from build123d import *

# Parameters (mm, degrees)
BASE_DEPTH                            = 5
ESQUISSE3_R                           = 2
ESQUISSE3_W                           = 65
ESQUISSE3_H                           = 30
PER_AGE_ROUES_ENCODEUSES_DEPTH        = 6
CONG_1_R                              = 3
PER_AGE_BILLES_PORTEUSES_REACH        = 7
ESQUISSE6_R                           = 2
ESQUISSE6_R_2                         = 11
PER_AGE_PROFIL_S_REACH                = 7
ESQUISSE8_R                           = 3
ESQUISSE15_R                          = 2.2
PER_AGE_BLOC_MOTEUR_DEPTH             = 5
ESQUISSE16_W                          = 65
ESQUISSE16_H                          = 38
ENL_V_MAT_EXTRU_1_DEPTH               = 6
ESQUISSE19_R                          = 1.75
PER_AGE_ACTIONNEUR_MAIN_DE_DIEU_DEPTH = 6


with BuildPart() as part:
    # Esquisse1 → Base (new body)
    with BuildSketch(Plane.XY):
        Polygon((0, 0), (-200, 0), (-224.748737342, 24.748737342), (-224.748737342, 284.748737342), (-200, 309.497474683), (0, 309.497474683), (24.748737342, 284.748737342), (24.748737342, 24.748737342), align=None)
    extrude(amount=BASE_DEPTH)

    # Esquisse3 → Perçage roues encodeuses (cut, through all)
    with BuildSketch(Plane(origin=(0, 0, 0), x_dir=(-1, 0, 0), z_dir=(0, 0, -1))):
        with Locations((65, 45)):
            Circle(ESQUISSE3_R)
        with Locations((135, 45)):
            Circle(ESQUISSE3_R)
        with Locations((135, 264.497474683)):
            Circle(ESQUISSE3_R)
        with Locations((65, 264.497474683)):
            Circle(ESQUISSE3_R)
        Polygon((142, 0), (142, 20), (118, 20), (118, 45.5), (82, 45.5), (82, 20), (58, 20), (58, 0), align=None)
        Polygon((58, 309.497474683), (142, 309.497474683), (142, 289.497474683), (118, 289.497474683), (118, 263.997474683), (82, 263.997474683), (82, 289.497474683), (58, 289.497474683), align=None)
        with Locations((100, 229.497474683)):
            Rectangle(ESQUISSE3_W, ESQUISSE3_H)
        with Locations((100, 80)):
            Rectangle(ESQUISSE3_W, ESQUISSE3_H)
    extrude(amount=-PER_AGE_ROUES_ENCODEUSES_DEPTH, mode=Mode.SUBTRACT)

    # Congé1
    cong_1_edges = [part.edges().sort_by_distance(p)[0] for p in [
        (0, 0, 2.5),
        (-200, 0, 2.5),
        (-224.748737342, 24.748737342, 2.5),
        (-224.748737342, 284.748737342, 2.5),
        (-200, 309.497474683, 2.5),
        (0, 309.497474683, 2.5),
        (24.748737342, 284.748737342, 2.5),
        (24.748737342, 24.748737342, 2.5),
        (-58, 289.497474683, 2.5),
        (-58, 309.497474683, 2.5),
        (-142, 309.497474683, 2.5),
        (-142, 289.497474683, 2.5),
        (-118, 289.497474683, 2.5),
        (-118, 263.997474683, 2.5),
        (-82, 263.997474683, 2.5),
        (-82, 289.497474683, 2.5),
        (-142, 0, 2.5),
        (-58, 0, 2.5),
        (-58, 20, 2.5),
        (-82, 20, 2.5),
        (-82, 45.5, 2.5),
        (-118, 45.5, 2.5),
        (-118, 20, 2.5),
        (-142, 20, 2.5),
    ]]
    fillet(cong_1_edges, radius=CONG_1_R)

    # Esquisse6 → Perçage billes porteuses (cut, up to next)
    with BuildSketch(Plane.XY.offset(5), mode=Mode.PRIVATE) as per_age_billes_porteuses_sk1:
        with Locations((-180.748737342, 28)):
            Circle(ESQUISSE6_R)
    per_age_billes_porteuses_tool1 = extrude(per_age_billes_porteuses_sk1.sketch, amount=-PER_AGE_BILLES_PORTEUSES_REACH, mode=Mode.PRIVATE) & part.part
    add(per_age_billes_porteuses_tool1.solids().sort_by_distance((-180.748737, 28, 5))[0], mode=Mode.SUBTRACT)
    # Esquisse6 → Perçage billes porteuses (cut, up to next)
    with BuildSketch(Plane.XY.offset(5), mode=Mode.PRIVATE) as per_age_billes_porteuses_sk2:
        with Locations((-210.748737342, 28)):
            Circle(ESQUISSE6_R)
    per_age_billes_porteuses_tool2 = extrude(per_age_billes_porteuses_sk2.sketch, amount=-PER_AGE_BILLES_PORTEUSES_REACH, mode=Mode.PRIVATE) & part.part
    add(per_age_billes_porteuses_tool2.solids().sort_by_distance((-210.748737, 28, 5))[0], mode=Mode.SUBTRACT)
    # Esquisse6 → Perçage billes porteuses (cut, up to next)
    with BuildSketch(Plane.XY.offset(5), mode=Mode.PRIVATE) as per_age_billes_porteuses_sk3:
        with Locations((-195.748737342, 28)):
            Circle(ESQUISSE6_R_2)
    per_age_billes_porteuses_tool3 = extrude(per_age_billes_porteuses_sk3.sketch, amount=-PER_AGE_BILLES_PORTEUSES_REACH, mode=Mode.PRIVATE) & part.part
    add(per_age_billes_porteuses_tool3.solids().sort_by_distance((-195.748737, 28, 5))[0], mode=Mode.SUBTRACT)
    # Esquisse6 → Perçage billes porteuses (cut, up to next)
    with BuildSketch(Plane.XY.offset(5), mode=Mode.PRIVATE) as per_age_billes_porteuses_sk4:
        with Locations((-19.251262658, 28)):
            Circle(ESQUISSE6_R)
    per_age_billes_porteuses_tool4 = extrude(per_age_billes_porteuses_sk4.sketch, amount=-PER_AGE_BILLES_PORTEUSES_REACH, mode=Mode.PRIVATE) & part.part
    add(per_age_billes_porteuses_tool4.solids().sort_by_distance((-19.251263, 28, 5))[0], mode=Mode.SUBTRACT)
    # Esquisse6 → Perçage billes porteuses (cut, up to next)
    with BuildSketch(Plane.XY.offset(5), mode=Mode.PRIVATE) as per_age_billes_porteuses_sk5:
        with Locations((10.748737342, 28)):
            Circle(ESQUISSE6_R)
    per_age_billes_porteuses_tool5 = extrude(per_age_billes_porteuses_sk5.sketch, amount=-PER_AGE_BILLES_PORTEUSES_REACH, mode=Mode.PRIVATE) & part.part
    add(per_age_billes_porteuses_tool5.solids().sort_by_distance((10.748737, 28, 5))[0], mode=Mode.SUBTRACT)
    # Esquisse6 → Perçage billes porteuses (cut, up to next)
    with BuildSketch(Plane.XY.offset(5), mode=Mode.PRIVATE) as per_age_billes_porteuses_sk6:
        with Locations((-4.251262658, 28)):
            Circle(ESQUISSE6_R_2)
    per_age_billes_porteuses_tool6 = extrude(per_age_billes_porteuses_sk6.sketch, amount=-PER_AGE_BILLES_PORTEUSES_REACH, mode=Mode.PRIVATE) & part.part
    add(per_age_billes_porteuses_tool6.solids().sort_by_distance((-4.251263, 28, 5))[0], mode=Mode.SUBTRACT)
    # Esquisse6 → Perçage billes porteuses (cut, up to next)
    with BuildSketch(Plane.XY.offset(5), mode=Mode.PRIVATE) as per_age_billes_porteuses_sk7:
        with Locations((-4.251262658, 281.497474683)):
            Circle(ESQUISSE6_R_2)
    per_age_billes_porteuses_tool7 = extrude(per_age_billes_porteuses_sk7.sketch, amount=-PER_AGE_BILLES_PORTEUSES_REACH, mode=Mode.PRIVATE) & part.part
    add(per_age_billes_porteuses_tool7.solids().sort_by_distance((-4.251263, 281.497475, 5))[0], mode=Mode.SUBTRACT)
    # Esquisse6 → Perçage billes porteuses (cut, up to next)
    with BuildSketch(Plane.XY.offset(5), mode=Mode.PRIVATE) as per_age_billes_porteuses_sk8:
        with Locations((10.748737342, 281.497474683)):
            Circle(ESQUISSE6_R)
    per_age_billes_porteuses_tool8 = extrude(per_age_billes_porteuses_sk8.sketch, amount=-PER_AGE_BILLES_PORTEUSES_REACH, mode=Mode.PRIVATE) & part.part
    add(per_age_billes_porteuses_tool8.solids().sort_by_distance((10.748737, 281.497475, 5))[0], mode=Mode.SUBTRACT)
    # Esquisse6 → Perçage billes porteuses (cut, up to next)
    with BuildSketch(Plane.XY.offset(5), mode=Mode.PRIVATE) as per_age_billes_porteuses_sk9:
        with Locations((-19.251262658, 281.497474683)):
            Circle(ESQUISSE6_R)
    per_age_billes_porteuses_tool9 = extrude(per_age_billes_porteuses_sk9.sketch, amount=-PER_AGE_BILLES_PORTEUSES_REACH, mode=Mode.PRIVATE) & part.part
    add(per_age_billes_porteuses_tool9.solids().sort_by_distance((-19.251263, 281.497475, 5))[0], mode=Mode.SUBTRACT)
    # Esquisse6 → Perçage billes porteuses (cut, up to next)
    with BuildSketch(Plane.XY.offset(5), mode=Mode.PRIVATE) as per_age_billes_porteuses_sk10:
        with Locations((-195.748737342, 281.497474683)):
            Circle(ESQUISSE6_R_2)
    per_age_billes_porteuses_tool10 = extrude(per_age_billes_porteuses_sk10.sketch, amount=-PER_AGE_BILLES_PORTEUSES_REACH, mode=Mode.PRIVATE) & part.part
    add(per_age_billes_porteuses_tool10.solids().sort_by_distance((-195.748737, 281.497475, 5))[0], mode=Mode.SUBTRACT)
    # Esquisse6 → Perçage billes porteuses (cut, up to next)
    with BuildSketch(Plane.XY.offset(5), mode=Mode.PRIVATE) as per_age_billes_porteuses_sk11:
        with Locations((-210.748737342, 281.497474683)):
            Circle(ESQUISSE6_R)
    per_age_billes_porteuses_tool11 = extrude(per_age_billes_porteuses_sk11.sketch, amount=-PER_AGE_BILLES_PORTEUSES_REACH, mode=Mode.PRIVATE) & part.part
    add(per_age_billes_porteuses_tool11.solids().sort_by_distance((-210.748737, 281.497475, 5))[0], mode=Mode.SUBTRACT)
    # Esquisse6 → Perçage billes porteuses (cut, up to next)
    with BuildSketch(Plane.XY.offset(5), mode=Mode.PRIVATE) as per_age_billes_porteuses_sk12:
        with Locations((-180.748737342, 281.497474683)):
            Circle(ESQUISSE6_R)
    per_age_billes_porteuses_tool12 = extrude(per_age_billes_porteuses_sk12.sketch, amount=-PER_AGE_BILLES_PORTEUSES_REACH, mode=Mode.PRIVATE) & part.part
    add(per_age_billes_porteuses_tool12.solids().sort_by_distance((-180.748737, 281.497475, 5))[0], mode=Mode.SUBTRACT)

    # Esquisse8 → Perçage profilés (cut, up to next)
    with BuildSketch(Plane.XY.offset(5), mode=Mode.PRIVATE) as per_age_profil_s_sk1:
        with Locations((-165, 23)):
            Circle(ESQUISSE8_R)
    per_age_profil_s_tool1 = extrude(per_age_profil_s_sk1.sketch, amount=-PER_AGE_PROFIL_S_REACH, mode=Mode.PRIVATE) & part.part
    add(per_age_profil_s_tool1.solids().sort_by_distance((-165, 23, 5))[0], mode=Mode.SUBTRACT)
    # Esquisse8 → Perçage profilés (cut, up to next)
    with BuildSketch(Plane.XY.offset(5), mode=Mode.PRIVATE) as per_age_profil_s_sk2:
        with Locations((-165, 286.497474683)):
            Circle(ESQUISSE8_R)
    per_age_profil_s_tool2 = extrude(per_age_profil_s_sk2.sketch, amount=-PER_AGE_PROFIL_S_REACH, mode=Mode.PRIVATE) & part.part
    add(per_age_profil_s_tool2.solids().sort_by_distance((-165, 286.497475, 5))[0], mode=Mode.SUBTRACT)
    # Esquisse8 → Perçage profilés (cut, up to next)
    with BuildSketch(Plane.XY.offset(5), mode=Mode.PRIVATE) as per_age_profil_s_sk3:
        with Locations((-35, 286.497474683)):
            Circle(ESQUISSE8_R)
    per_age_profil_s_tool3 = extrude(per_age_profil_s_sk3.sketch, amount=-PER_AGE_PROFIL_S_REACH, mode=Mode.PRIVATE) & part.part
    add(per_age_profil_s_tool3.solids().sort_by_distance((-35, 286.497475, 5))[0], mode=Mode.SUBTRACT)
    # Esquisse8 → Perçage profilés (cut, up to next)
    with BuildSketch(Plane.XY.offset(5), mode=Mode.PRIVATE) as per_age_profil_s_sk4:
        with Locations((-35, 23)):
            Circle(ESQUISSE8_R)
    per_age_profil_s_tool4 = extrude(per_age_profil_s_sk4.sketch, amount=-PER_AGE_PROFIL_S_REACH, mode=Mode.PRIVATE) & part.part
    add(per_age_profil_s_tool4.solids().sort_by_distance((-35, 23, 5))[0], mode=Mode.SUBTRACT)

    # Esquisse15 → Perçage bloc moteur (cut)
    with BuildSketch(Plane(origin=(0, 0, 0), x_dir=(-1, 0, 0), z_dir=(0, 0, -1))):
        with Locations((114, 103)):
            Circle(ESQUISSE15_R)
        with Locations((32, 103)):
            Circle(ESQUISSE15_R)
        with Locations((114, 57)):
            Circle(ESQUISSE15_R)
        with Locations((32, 57)):
            Circle(ESQUISSE15_R)
        with Locations((32, 252.497474683)):
            Circle(ESQUISSE15_R)
        with Locations((114, 252.497474683)):
            Circle(ESQUISSE15_R)
        with Locations((114, 206.497474683)):
            Circle(ESQUISSE15_R)
        with Locations((32, 206.497474683)):
            Circle(ESQUISSE15_R)
    extrude(amount=-PER_AGE_BLOC_MOTEUR_DEPTH, mode=Mode.SUBTRACT)

    # Esquisse16 → Enlèv. mat.-Extru.1 (cut, through all)
    with BuildSketch(Plane(origin=(0, 0, 0), x_dir=(-1, 0, 0), z_dir=(0, 0, -1))):
        with Locations((100, 80)):
            Rectangle(ESQUISSE16_W, ESQUISSE16_H)
        with Locations((100, 229.497474683)):
            Rectangle(ESQUISSE16_W, ESQUISSE16_H)
    extrude(amount=-ENL_V_MAT_EXTRU_1_DEPTH, mode=Mode.SUBTRACT)

    # Esquisse19 → Perçage actionneur Main_De_Dieu (cut, through all)
    with BuildSketch(Plane(origin=(0, 0, 0), x_dir=(-1, 0, 0), z_dir=(0, 0, -1))):
        with Locations((166.148737342, 137.798737342)):
            Circle(ESQUISSE19_R)
        with Locations((174.148737342, 137.798737342)):
            Circle(ESQUISSE19_R)
        with Locations((-7.248737342, 231.748737342)):
            Circle(ESQUISSE19_R)
        with Locations((12.751262658, 231.748737342)):
            Circle(ESQUISSE19_R)
        with Locations((12.751262658, 77.748737342)):
            Circle(ESQUISSE19_R)
        with Locations((-7.248737342, 77.748737342)):
            Circle(ESQUISSE19_R)
        with Locations((187.248737342, 77.748737342)):
            Circle(ESQUISSE19_R)
        with Locations((207.248737342, 77.748737342)):
            Circle(ESQUISSE19_R)
        with Locations((207.248737342, 231.748737342)):
            Circle(ESQUISSE19_R)
        with Locations((187.248737342, 231.748737342)):
            Circle(ESQUISSE19_R)
        with Locations((25.851262658, 171.698737342)):
            Circle(ESQUISSE19_R)
        with Locations((33.851262658, 171.698737342)):
            Circle(ESQUISSE19_R)
    extrude(amount=-PER_AGE_ACTIONNEUR_MAIN_DE_DIEU_DEPTH, mode=Mode.SUBTRACT)


solid = part.part
Design review of the part built by this model. Coordinates are the model's own, in mm. Coordinates: 2 decimals unless noted, no trailing zeros. Order: outer loops, then holes, each group sorted by start corner. A loop starts at its lowest first (then second) coordinate and runs counter-clockwise, first axis right, second up. Notation, with made-up numbers: (-5.5, 47) -> (19.5, 47) arc R16 ccw to (19.5, 75) -> close; hole circle Ø6 at (-1, 24.5). An arc over 180 degrees is marked (long way). Use one line per item in the form item = value. Start each with the question number.
(1) The part is to be moulded in two halves that separate along X. For faces 1 (the flat face through (-98, 157, 5)), 2 (the flat face through (13, 13, 2)), 3 (the cylindrical face through (-185.588, 23.787, 2.535)), say which applies: +X half, -X half, draft (parallel to the pull), parting line (faces both ways), or undercut.
(2) For probe 1 along X at (y, z) = (138, 1.5); probe 2 along Y at (x, z) = (-65, 0.65); probe 3 along X at (y, z) = (24.5, 3.4), list the stretches that pass through material, from the lowest coordinate up.
(3) Add section B-B on z = 1.2. Give the number of separate pieces and of enclosed holes in the cut face, plus the area to 3 significant figures.
(4) Insertion check: pin 1 (2.5 mm diameter, centred on y = 11.5, z = 3, fed in from +X); pin 2 (1.5 mm diameter, centred on y = 11, z = 2, fed in from -X); pin 3 (1.5 mm diameter, centred on x = -99, z = 2.5, fed in from +Y). Each pin has a flat end and moves straight along its axis. Give the tip position at first contact, or say it passes through.
(5) Add section A-A on x = -124.5. State the section outline as (y, z) points.
Answer block:
q1.face_1 = draft
q1.face_2 = +X half
q1.face_3 = undercut
q2.probe_1 = -224.75 to -175.89, -172.41 to -167.89, -164.41 to 24.75
q2.probe_2 = 20 to 43, 47 to 262.5, 266.5 to 289.5
q2.probe_3 = -224.35 to -206.18, -185.32 to -167.6, -162.4 to -118, -82 to -37.6, -32.4 to -14.68, 6.18 to 24.35
q3.separate_pieces = 1
q3.enclosed_holes = 42
q3.area = 63,800 mm²
q4.pin_1 = 12.75
q4.pin_2 = -211.75
q4.pin_3 = 264
q5.outline = (20, 0) -> (61, 0) -> (61, 5) -> (20, 5) -> close; (99, 0) -> (210.5, 0) -> (210.5, 5) -> (99, 5) -> close; (248.5, 0) -> (289.5, 0) -> (289.5, 5) -> (248.5, 5) -> close
